Geometry check sheet. Reference: the model listing, model coordinates, mm. A direction names the side the tool comes from. Coordinates: 2 decimals unless noted, no trailing zeros. Write each loop counter-clockwise with the first axis right and the second up, starting at its lowest first coordinate (ties: lowest second). Pieces come first, ordered by that corner, then holes.
from build123d import *

# Parameters (mm, degrees)
SKETCH1_W           = 177
SKETCH1_H           = 99
SKETCH1_H_2         = 42
SKETCH1_W_2         = 220
SKETCH1_H_3         = 160
SKETCH1_W_3         = 89
SKETCH1_W_4         = 99
SKETCH1_W_5         = 137
SKETCH1_H_4         = 254
SKETCH1_W_6         = 59
BOSS_EXTRUDE1_DEPTH = 19


with BuildPart() as part:
    # Sketch1 → Boss-Extrude1 (new body)
    with BuildSketch(Plane(origin=(0, 0, 0), x_dir=(1, 0, 0), z_dir=(0, 1, 0))):
        Polygon((-340, 325), (-340, -325), (340, -325), (340, 325), (125, 325), (125, 146), (-125, 146), (-125, 325), align=None)
        with Locations((-232.5, -256.5)):
            Rectangle(SKETCH1_W, SKETCH1_H, mode=Mode.SUBTRACT)
        with Locations((-232.5, -167)):
            Rectangle(SKETCH1_W, SKETCH1_H_2, mode=Mode.SUBTRACT)
        with Locations((-15, -226)):
            Rectangle(SKETCH1_W_2, SKETCH1_H_3, mode=Mode.SUBTRACT)
        with Locations((158.5, -226)):
            Rectangle(SKETCH1_W_3, SKETCH1_H_3, mode=Mode.SUBTRACT)
        with Locations((271.5, -226)):
            Rectangle(SKETCH1_W_4, SKETCH1_H_3, mode=Mode.SUBTRACT)
        with Locations((-252.5, 0)):
            Rectangle(SKETCH1_W_5, SKETCH1_H_4, mode=Mode.SUBTRACT)
        with Locations((-271.5, 226)):
            Rectangle(SKETCH1_W_4, SKETCH1_H_3, mode=Mode.SUBTRACT)
        with Locations((-173.5, 226)):
            Rectangle(SKETCH1_W_6, SKETCH1_H_3, mode=Mode.SUBTRACT)
        Polygon((-165, -127), (-165, 127), (132.861538462, 127), (165, 127), (165, -127), (114, -127), (95, -127), (-125, -127), (-144, -127), align=None, mode=Mode.SUBTRACT)
        with Locations((252.5, 0)):
            Rectangle(SKETCH1_W_5, SKETCH1_H_4, mode=Mode.SUBTRACT)
        with Locations((232.5, 167)):
            Rectangle(SKETCH1_W, SKETCH1_H_2, mode=Mode.SUBTRACT)
        with Locations((232.5, 256.5)):
            Rectangle(SKETCH1_W, SKETCH1_H, mode=Mode.SUBTRACT)
    extrude(amount=BOSS_EXTRUDE1_DEPTH)


solid = part.part
1. Access from +Z, -Z, +X, -X, +Y, -Y to the whole of each face (thin tool, end or side, straight path). Record for faces 3 (the flat face through (24, 0, 143)), 4 (the flat face through (321, 9, 227)), 5 (the flat face through (125, 9, -237)).
Computed values:
face 3: +Z, -Z, +X, -X, -Y
face 4: +Y, -Y
face 5: -Z, +Y, -Y
2. Draft check along Z on faces 1 (the flat face through (-125, 9, -234)), 2 (the flat face through (158, 9, 306)). Enter one of: released by +Z, released by -Z, zero draft, split by the parting line, or undercut.
Computed values:
face 1: zero draft
face 2: undercut
3. Gauge pin test, flat end, axial feed: pin 1 Ø2 at (x, y) = (-98, 10) entering from -Z. Record the tip position at first contact, or that the pin passes through.
Computed values:
pin 1: stops at z = -146
4. Sectioned sample at B-B, the plane z = 282. Record the boundary of the cut face in (x, y), and give its area (4 significant figures).
Computed values:
outline: (-340, 0) - (-321, 0) - (-321, 19) - (-340, 19) - close; (-144, 0) - (-125, 0) - (-125, 19) - (-144, 19) - close; (95, 0) - (114, 0) - (114, 19) - (95, 19) - close; (203, 0) - (222, 0) - (222, 19) - (203, 19) - close; (321, 0) - (340, 0) - (340, 19) - (321, 19) - close
area: 1,805 mm2
5. Sectioned sample at A-A, the plane x = 257. Record the boundary of the cut face in (y, z).
Computed values:
outline: (0, -325) - (19, -325) - (19, -306) - (0, -306) - close; (0, -207) - (19, -207) - (19, -188) - (0, -188) - close; (0, -146) - (19, -146) - (19, -127) - (0, -127) - close; (0, 127) - (19, 127) - (19, 146) - (0, 146) - close; (0, 306) - (19, 306) - (19, 325) - (0, 325) - close
6. Sectioned sample at D-D, the plane z = -94. Record the boundary of the cut face in (x, y), and give its area (3 significant figures).
Computed values:
outline: (-340, 0) - (-321, 0) - (-321, 19) - (-340, 19) - close; (-184, 0) - (-165, 0) - (-165, 19) - (-184, 19) - close; (165, 0) - (184, 0) - (184, 19) - (165, 19) - close; (321, 0) - (340, 0) - (340, 19) - (321, 19) - close
area: 1,440 mm2
7. Thickness scan on line 1 along Z through (x, y) = (-97, 14.5); line 2 along Z through (x, y) = (-308.5, 10.75); line 3 along X through (y, z) = (6.75, -181). Record the ranges inside material, lowest first.
Computed values:
line 1: z = -146 to -127, 127 to 146, 306 to 325
line 2: z = -325 to -306, -146 to -127, 127 to 146, 188 to 207, 306 to 325
line 3: x = -340 to -321, -222 to -203, -144 to -125, 125 to 144, 321 to 340
8. Sectioned sample at C-C, the plane x = -97. Record the boundary of the cut face in (y, z).
Computed values:
outline: (0, -146) - (19, -146) - (19, -127) - (0, -127) - close; (0, 127) - (19, 127) - (19, 146) - (0, 146) - close; (0, 306) - (19, 306) - (19, 325) - (0, 325) - close
